Build history of the part. All positions in model axes, mm. A direction names the side the tool comes from. Round coordinates to 2 decimals unless told otherwise and drop trailing zeros. Order: outer loops, then holes, each group sorted by start corner. A loop starts at its lowest first (then second) coordinate and runs counter-clockwise, first axis right, second up. Notation, with made-up numbers: M -33.75,15 L 16.25,15 A29 ccw 16.25,38 Z; hole C 32.5,-11 d4. An arc over 180 degrees is marked long. One line per item, written item: value. Start each with the question number.
Item 1: Band-saw the part on A-A, the plane z = 5. Write the cut outline in (x, y), then the cut area to 3 significant figures.
Item 2: Two-plate mould, pull along X, no slides. Class faces 3 (the flat face through (242, 2, 61.4)), 4 (the cylindrical face through (241.863, 2.117, 4.31)), 5 (the cylindrical face through (245.477, 4.098, 30.524)), 6 (the conical face through (240.548, 2.743, 55.779)): +X half, -X half, draft (parallel to the pull), parting line (faces both ways), or undercut.
Item 3: Tool access for faces 1 (the cylindrical face through (239.554, 2.117, 58.865)), 2 (the flat face through (242, 2, 0)): list every direction of +Z, -Z, +X, -X, +Y, -Y with a clear straight run to the whole face (end or side of a thin tool).
Item 4: Band-saw the part on B-B, the plane z = 28. Write the cut outline in (x, y), then the cut area to 3 significant figures.
Item 5: Probe L1, parallel to Y at x = 240.5, z = 29; L2, parallel to Z at x = 242.25, y = -1.75; L3, parallel to X at y = 2.5, z = 17. List the from-to ranges inside material, lowest first.
Item 6: Pin check, flat tips, straight feed: pin 1 (1.5 mm diameter, centred on x = 240.71, y = 2.6, fed in from +Z); pin 2 (5 mm diameter, centred on x = 244.5, z = 47, fed in from +Y); pin 3 (1 mm diameter, centred on x = 244.5, z = 35.5, fed in from -Y). Stop position of each tip, or through.
```python
from build123d import *

# Parameters (mm, degrees)
ESBO_O1_R                                      = 5
RESSALTO_EXTRUS_O1_DEPTH                       = 61.4
FURO_ROSCADO_DE_M3X0_52_D                      = 2.5
FURO_ROSCADO_DE_M3X0_52_DEPTH                  = 8.5
FURO_ROSCADO_DE_M3X0_52_TIP                    = 0.751075774
FILETE1_R                                      = 0.5
BROCA_DE_ROSQUEAR_PARA_TARRAXA_DE_M3X0_5_D     = 2.5
BROCA_DE_ROSQUEAR_PARA_TARRAXA_DE_M3X0_5_DEPTH = 5
BROCA_DE_ROSQUEAR_PARA_TARRAXA_DE_M3X0_5_TIP   = 0.751075774


with BuildPart() as part:
    # Esboço1 → Ressalto-extrusão1 (new body)
    with BuildSketch(Plane.XY):
        with Locations((240.708388302, 2.596082859)):
            Circle(ESBO_O1_R)
    extrude(amount=RESSALTO_EXTRUS_O1_DEPTH)

    # Furo roscado de M3x0.52
    with Locations(Plane(origin=(0, 0, 0), x_dir=(-1, 0, 0), z_dir=(0, 0, -1))):
        with Locations((-240.708388302, 2.596082859)):
            Hole(FURO_ROSCADO_DE_M3X0_52_D / 2, depth=FURO_ROSCADO_DE_M3X0_52_DEPTH)
            with Locations((0, 0, -(FURO_ROSCADO_DE_M3X0_52_DEPTH + FURO_ROSCADO_DE_M3X0_52_TIP / 2))):  # 118° drill point
                Cone(0, FURO_ROSCADO_DE_M3X0_52_D / 2, FURO_ROSCADO_DE_M3X0_52_TIP, mode=Mode.SUBTRACT)

    # Filete1
    filete1_edges = [part.edges().sort_by_distance(p)[0] for p in [
        (235.708388302, 2.596082859, 0),
    ]]
    fillet(filete1_edges, radius=FILETE1_R)

    # Broca de rosquear para tarraxa de M3x0.51
    with Locations(Plane.XY.offset(61.4)):
        with Locations((240.708388302, 2.596082859)):
            Hole(BROCA_DE_ROSQUEAR_PARA_TARRAXA_DE_M3X0_5_D / 2, depth=BROCA_DE_ROSQUEAR_PARA_TARRAXA_DE_M3X0_5_DEPTH)
            with Locations((0, 0, -(BROCA_DE_ROSQUEAR_PARA_TARRAXA_DE_M3X0_5_DEPTH + BROCA_DE_ROSQUEAR_PARA_TARRAXA_DE_M3X0_5_TIP / 2))):  # 118° drill point
                Cone(0, BROCA_DE_ROSQUEAR_PARA_TARRAXA_DE_M3X0_5_D / 2, BROCA_DE_ROSQUEAR_PARA_TARRAXA_DE_M3X0_5_TIP, mode=Mode.SUBTRACT)


solid = part.part
```
Output:
1. outline: C 240.71,2.6 d10; hole C 240.71,2.6 d2.5
1. area: 73.6 mm²
2. face 3: draft
2. face 4: undercut
2. face 5: parting line
2. face 6: undercut
3. face 1: +Z
3. face 2: -Z, +X, -X, +Y, -Y
4. outline: C 240.71,2.6 d10
4. area: 78.5 mm²
5. L1: y = -2.4 to 7.59
5. L2: z = 0.01 to 61.4
5. L3: x = 235.71 to 245.71
6. pin 1: stops at z = 56.1
6. pin 2: stops at y = 7.43
6. pin 3: stops at y = -1.17
